```python
from build123d import *

# Parameters (mm, degrees)
F1_DEPTH = 62
F2_R     = 10
F3_R     = 5
F4_R     = 5
F6_DEPTH = 666
F7_R     = 15.99999
F8_R     = 8
F9_DEPTH = 25


# Not quite as in the source:
# - a fillet or chamfer is up to 0.001 mm smaller than in the source, because OpenCascade refuses the exact size


with BuildPart() as f1:
    # F0 (on Front) → F1 (new body)
    with BuildSketch(Plane.XZ):
        Polygon((-76, 67.66280128), (-90, 67.66280128), (-90, 32.66280128), (0, 32.66280128), (0, 8.0000054104), (20, 8.0000054104), (20, 46.66280128), (-76, 46.66280128), align=None)
    extrude(amount=F1_DEPTH)

    # F2
    f2_edges = [f1.edges().sort_by_distance(p)[0] for p in [
        (-83, -62, 67.662801),
        (-83, 0, 67.662801),
    ]]
    fillet(f2_edges, radius=F2_R)

    # F3
    f3_edges = [f1.edges().sort_by_distance(p)[0] for p in [
        (-76, -31, 46.662801),
    ]]
    fillet(f3_edges, radius=F3_R)

    # F4
    f4_edges = [f1.edges().sort_by_distance(p)[0] for p in [
        (0, -31, 32.662801),
    ]]
    fillet(f4_edges, radius=F4_R)

    # F5 (on face) → F6 (cut)
    with BuildSketch(Plane.XY.offset(46.66280128)):
        Polygon((20, -62), (20, -47), (-15.907, -47), (-30.907, -62), align=None)
        Polygon((-15.907, -15), (20, -15), (20, 0), (-30.907, 0), align=None)
    extrude(amount=-F6_DEPTH, mode=Mode.SUBTRACT)

    # F7 (radius 16 in the source; OpenCascade refuses exactly that, so slightly less here)
    f7_edges = [f1.edges().sort_by_distance(p)[0] for p in [
        (10, -47, 8.000005),
        (10, -15, 8.000005),
    ]]
    fillet(f7_edges, radius=F7_R)

    # F8 (on face) → F9 (cut)
    with BuildSketch(Plane.YZ.offset(20)):
        with Locations((-31, 24.0000054104)):
            Circle(F8_R)
    extrude(amount=-F9_DEPTH, mode=Mode.SUBTRACT)


solid = f1.part
```
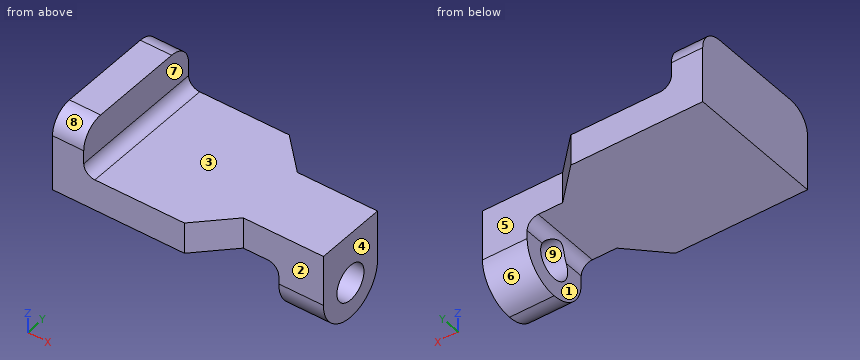
Geometry check sheet. Reference: the model listing, model coordinates, mm. Face numbers are marked on the shaded views. A direction names the side the tool comes from. Round coordinates to 2 decimals unless told otherwise and drop trailing zeros. Order: outer loops, then holes, each group sorted by start corner. A loop starts at its lowest first (then second) coordinate and runs counter-clockwise, first axis right, second up. Notation, with made-up numbers: (-15.75, 5) - (22.25, 5) arc R20 cw to (22.25, 32) - close; hole circle Ø5 at (35, 38). An arc over 180 degrees is marked (long way). Use a Markdown table: item, result. Add a question column.
(1) Tool access check on the marked faces 1, 2, 3, 4 and 5. Record the directions out of +Z, -Z, +X, -X, +Y, -Y that give a thin tool (end or side, any length) a straight path to the whole face; none if there is none.
(2) Sectioned sample at B-B, the plane z = 21.5. Enter the section's corners in (x, y), and give its area (3 significant figures).
(3) Sectioned sample at D-D, the plane y = -13.5. Enter the section's corners in (x, z), and give its area (3 significant figures).
(4) Sectioned sample at C-C, the plane z = 36. Enter the section's corners in (x, y).
(5) Material ranges on line 1 along Z through (x, y) = (15, -31); line 2 along Z through (x, y) = (-82, -12); line 3 along X through (y, z) = (-8.5, 61), recorded low to high. Write a range as [from, to].
(6) Depth check by flat-ended pin: pin 1 (6 mm diameter, centred on x = 6, z = 23.5, fed in from +Y); pin 2 (18.5 mm diameter, centred on x = -63, y = -17.5, fed in from -Z); pin 3 (13 mm diameter, centred on y = -38.5, z = 59.5, fed in from +X). Enter the tip coordinate at first touch or a pass-through.
(7) Release check for a two-part mould opening along Z. For the marked faces 6, 7, 8 and 9 record: pulls with the +Z half, pulls with the -Z half, needs draft (parallel to the pull), parting line crosses it, or undercut.
Answers below:
| question | item | result |
|---|---|---|
| 1 | face 1 | -Z, -X, +Y, -Y |
| 1 | face 2 | +Z, -Z, +X, -Y |
| 1 | face 3 | +Z, +X, +Y, -Y |
| 1 | face 4 | +Z, -Z, +X, +Y, -Y |
| 1 | face 5 | +Z, -Z, +X, +Y |
| 2 | outline | (0, -46.8) - (20, -46.8) - (20, -38.6) - (0, -38.6) - close; (0, -23.4) - (20, -23.4) - (20, -15.2) - (0, -15.2) - close |
| 2 | area | 328 mm² |
| 3 | outline | (-90, 32.66) - (-17.41, 32.66) - (-17.41, 46.66) - (-71, 46.66) arc R5 cw to (-76, 51.66) - (-76, 67.66) - (-90, 67.66) - close |
| 3 | area | 1,320 mm² |
| 4 | outline | (-90, -62) - (-30.91, -62) - (-15.91, -47) - (20, -47) - (20, -15) - (-15.91, -15) - (-30.91, 0) - (-90, 0) - close |
| 5 | line 1 | [8, 16], [32, 46.66] |
| 5 | line 2 | [32.66, 67.66] |
| 5 | line 3 | [-90, -76] |
| 6 | pin 1 | y = -15 |
| 6 | pin 2 | z = 32.66 |
| 6 | pin 3 | x = -76 |
| 7 | face 6 | pulls with the -Z half |
| 7 | face 7 | needs draft |
| 7 | face 8 | pulls with the +Z half |
| 7 | face 9 | undercut |
